from build123d import *

# Parameters (mm, degrees)
F0_W      = 159
F0_H      = 129
F1_DEPTH  = 60
F2_R      = 5
F3_W      = 7.5
F3_H      = 93
F3_W_2    = 95
F3_H_2    = 11
F4_DEPTH  = 97
F5_R      = 5
F6_R      = 1
F7_T      = -1
F9_D      = 3.505
F10_R     = 10
F11_DEPTH = 10


with BuildPart() as f1:
    # F0 (on Front) → F1 (new body)
    with BuildSketch(Plane.XZ):
        with Locations((5.1108691841, -2.7578008189)):
            Rectangle(F0_W, F0_H)
    extrude(amount=F1_DEPTH)

    # F2
    f2_edges = [f1.edges().sort_by_distance(p)[0] for p in [
        (84.610869, -30, -67.257801),
        (84.610869, -30, 61.742199),
        (-74.389131, -30, 61.742199),
        (-74.389131, -30, -67.257801),
    ]]
    fillet(f2_edges, radius=F2_R)

    # F3 (on face) → F4 (cut)
    with BuildSketch(Plane.XZ.offset(60)):
        with Locations((-37.1391308159, -2.7578008189)):
            Rectangle(F3_W, F3_H)
        with Locations((14.1108691841, -2.7578008189)):
            Rectangle(F3_W_2, F3_H)
        with Locations((14.1108691841, 49.2421991811)):
            Rectangle(F3_W_2, F3_H_2)
        with Locations((65.3608691841, -2.7578008189)):
            Rectangle(F3_W, F3_H)
        with Locations((14.1108691841, -54.7578008189)):
            Rectangle(F3_W_2, F3_H_2)
    extrude(amount=-F4_DEPTH, mode=Mode.SUBTRACT)

    # F5
    f5_edges = [f1.edges().sort_by_distance(p)[0] for p in [
        (-33.389131, -30, 54.742199),
        (61.610869, -30, 54.742199),
        (61.610869, -30, -60.257801),
        (-33.389131, -30, -60.257801),
    ]]
    fillet(f5_edges, radius=F5_R)

    # F6
    f6_edges = [f1.edges().sort_by_distance(p)[0] for p in [
        (-33.389131, -30, 43.742199),
        (61.610869, -30, 43.742199),
        (61.610869, -30, -49.257801),
        (-33.389131, -30, -49.257801),
    ]]
    fillet(f6_edges, radius=F6_R)

    # F7
    f7_openings = [f1.faces().sort_by_distance(p)[0] for p in [
        (-37.639131, -30, 43.742199),
        (-33.389131, -30, 47.242199),
        (-31.924665, -30, 53.277733),
        (14.110869, -30, 54.742199),
        (60.146403, -30, 53.277733),
        (61.610869, -30, 47.242199),
        (65.860869, -30, 43.742199),
        (69.110869, -30, -2.757801),
        (65.860869, -30, -49.257801),
        (61.610869, -30, -52.757801),
        (60.146403, -30, -58.793335),
        (14.110869, -30, -60.257801),
        (-31.924665, -30, -58.793335),
        (-33.389131, -30, -52.757801),
        (-37.639131, -30, -49.257801),
        (-40.889131, -30, -2.757801),
        (-33.682024, -30, 44.035092),
        (61.903762, -30, 44.035092),
        (61.903762, -30, -49.550694),
        (-33.682024, -30, -49.550694),
    ]]
    offset(amount=F7_T, openings=f7_openings)

    # F9 (through all)
    with Locations(Plane.XZ.offset(60)):
        with Locations((-38.8891308159, 49.7421991811), (66.1108691841, 49.7421991811), (66.1108691841, -55.2578008189), (-38.8891308159, -55.2578008189)):
            Hole(F9_D / 2)

    # F10 (on face) → F11 (cut)
    with BuildSketch(Plane.XZ.offset(60)):
        with Locations((-61.3891308159, 29.2421991811)):
            Circle(F10_R)
        with Locations((-61.3891308159, -34.7578008189)):
            Circle(F10_R)
    extrude(amount=-F11_DEPTH, mode=Mode.SUBTRACT)


solid = f1.part
Here's how the part is built. I have some questions about the finished solid (model axes, mm). A direction names the side the tool comes from. Round coordinates to 2 decimals unless told otherwise and drop trailing zeros. Loops run counter-clockwise (first coordinate to the right, second up) from the corner with the lowest first, then second, coordinate; pieces in that order, holes last. Notation, with made-up numbers: M -15,73 L 1,73 A26 ccw 1,111 Z; hole C 9.5,-18 d10. An arc over 180 degrees is marked long. Write each question's results on one line, items separated by ' | '. Start each with the question number.
(1) I want a section at A-A (z = -12). Please give me the cut outline in (x, y).
(2) I want a section at D-D (y = -25). Please give me the cut outline in (x, z), then the cut area to 3 significant figures.
(3) On a 3-axis mill with a long thin cutter (end or side, diameter ignored), from which of +Z, -Z, +X, -X, +Y, -Y can I reach the whole of each face in a straight line? I mean faces 5 (the cylindrical face through (-31.9, -59.5, 53.3)), 6 (the cylindrical face through (-69.325, -59.507, -40.843)), 7 (the flat face through (4, -30, -66.258)), 8 (the flat face through (-74.389, -30, -4)). Say none if no direction works.
(4) Will this pin go through, and if not, where does the flat tip stop? P1, Ø3, axis at x = -38.89, z = -55.26, coming from the +Y side.
(5) I want a section at B-B (x = 23.5). Please give me the cut outline in (y, z), then the cut area to 3 significant figures.
(6) Thinking about a two-plate mould opening in Z: for faces 1 (the cylindrical face through (-69.325, -59.507, 23.157)), 2 (the cylindrical face through (-72.963, -30.42, -65.754)), 3 (the flat face through (84.611, -30, -4)), 4 (the cylindrical face through (-72.25, -30.41, 59.54)), which applies, pulls with the +Z half, pulls with the -Z half, needs draft (parallel to the pull), parting line crosses it, or undercut?
(7) If I drill on probe 1 along Z at (x, y) = (52, -11.5); probe 2 along X at (y, z) = (-35.5, -50); probe 3 along Y at (x, z) = (-50.5, 45.5), over which ranges is the centre line in solid material (lowest first)? Write a range as from..to.
(8) I want a section at C-C (z = 26). Please give me the cut outline in (x, y), then the cut area to 3 significant figures.
Solved:
1) outline: M -74.39,-60 L -40.89,-60 L -40.89,-59 L -73.39,-59 L -73.39,-1 L -40.89,-1 L -40.89,0 L -74.39,0 Z; M 69.11,-60 L 84.61,-60 L 84.61,0 L 69.11,0 L 69.11,-1 L 83.61,-1 L 83.61,-59 L 69.11,-59 Z
2) outline: M -74.39,-62.26 A5 ccw -69.39,-67.26 L 79.61,-67.26 A5 ccw 84.61,-62.26 L 84.61,56.74 A5 ccw 79.61,61.74 L -69.39,61.74 A5 ccw -74.39,56.74 Z; hole M -73.39,-62.26 A4 ccw -69.39,-66.26 L 79.61,-66.26 A4 ccw 83.61,-62.26 L 83.61,56.74 A4 ccw 79.61,60.74 L -69.39,60.74 A4 ccw -73.39,56.74 Z | area: 564 mm²
3) face 5: +Y, -Y | face 6: -Y | face 7: none | face 8: +Z, -Z, -X, +Y, -Y
4) P1: passes through
5) outline: M -60,-67.26 L 0,-67.26 L 0,-60.26 L -1,-60.26 L -1,-66.26 L -59,-66.26 L -59,-60.26 L -60,-60.26 Z; M -60,54.74 L -59,54.74 L -59,60.74 L -1,60.74 L -1,54.74 L 0,54.74 L 0,61.74 L -60,61.74 Z | area: 144 mm²
6) face 1: undercut | face 2: pulls with the -Z half | face 3: needs draft | face 4: undercut
7) probe 1: z = -67.26..-66.26, 60.74..61.74 | probe 2: x = -74.39..-73.39, 83.61..84.61 | probe 3: y = -60..-59, -1..0
8) outline: M -74.39,-60 L -70.85,-60 L -70.85,-59 L -73.39,-59 L -73.39,-1 L -40.89,-1 L -40.89,0 L -74.39,0 Z; M -51.93,-60 L -40.89,-60 L -40.89,-59 L -51.93,-59 Z; M 69.11,-60 L 84.61,-60 L 84.61,0 L 69.11,0 L 69.11,-1 L 83.61,-1 L 83.61,-59 L 69.11,-59 Z | area: 195 mm²
